Geometry check sheet. Reference: the model listing, model coordinates, mm. Face numbers are marked on the shaded views. A direction names the side the tool comes from. Round coordinates to 2 decimals unless told otherwise and drop trailing zeros. Write each loop counter-clockwise with the first axis right and the second up, starting at its lowest first coordinate (ties: lowest second). Pieces come first, ordered by that corner, then holes. Notation, with made-up numbers: (75, -23) -> (129, -23) arc R20 ccw to (129, 9) -> close; hole circle Ø9 at (59.5, 30). An arc over 180 degrees is marked (long way). Use a Markdown table: item, result.
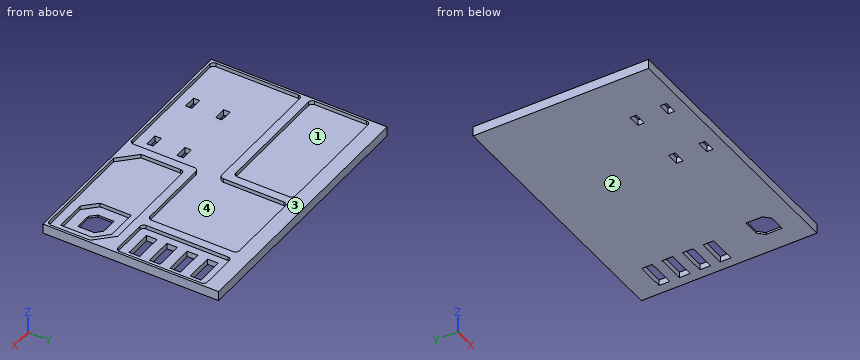
Autodesk Fusion 360 part; units mm, degrees
sketch "Sketch1" plane through (0, 0, 0) normal (0, 0, 1) x (1, 0, 0)
  line L0 (0, 0) -> (70.4, 0)
  line L1 (70.4, 0) -> (70.4, 46.4)
  line L2 (70.4, 46.4) -> (0, 46.4)
  line L3 (0, 46.4) -> (0, 0)
  line L4 (1.1, 1.1) -> (69.3, 1.1) construction
  line L5 (69.3, 1.1) -> (69.3, 45.3) construction
  line L6 (69.3, 45.3) -> (1.1, 45.3) construction
  line L7 (1.1, 45.3) -> (1.1, 1.1) construction
  line L8 (35.2, 45.3) -> (35.2, 1.1) construction
  line L9 (1.1, 23.2) -> (35.2, 23.2) construction
  line L10 (35.2, 23.2) -> (69.3, 23.2) construction
  line L11 (35.2, 45.3) -> (35.2, 42) construction
  line L12 (35.2, 42) -> (35, 42) construction
  line L13 (35, 42) -> (1.1, 42) construction
  line L14 (35.2, 42) -> (69.3, 42) construction
  line L15 (68.3, 42) -> (59.3, 42)
  line L16 (58.3, 41) -> (58.3, 19.9)
  line L17 (59.3, 18.9) -> (68.3, 18.9)
  line L18 (69.3, 19.9) -> (69.3, 41)
  line L19 (58.3, 30.45) -> (56.1, 30.45) construction
  line L20 (36.2, 42) -> (55.1, 42)
  line L21 (56.1, 41) -> (56.1, 19.9)
  line L22 (55.1, 18.9) -> (36.2, 18.9)
  line L23 (35.2, 30.45) -> (33, 30.45) construction
  line L24 (2.1, 42) -> (32, 42)
  line L25 (33, 41) -> (33, 27.6)
  line L26 (32, 26.6) -> (2.1, 26.6)
  line L27 (1.1, 27.6) -> (1.1, 41)
  line L28 (17.05, 26.6) -> (17.05, 24.4) construction
  line L29 (45.65, 18.9) -> (45.65, 16.7) construction
  line L30 (2.1, 1.1) -> (34.2, 1.1)
  line L31 (34.2, 24.3632) -> (2.1, 24.3632)
  line L32 (1.1, 23.3632) -> (1.1, 2.1)
  line L33 (35.2, 41) -> (35.2, 25.3632)
  line L34 (35.2, 17.9) -> (35.2, 2.1)
  line L35 (18.15, 24.3632) -> (18.15, 17.7632) construction
  line L36 (1.1, 1.1) -> (1.1, 2.2) construction
  line L37 (1.1, 1.1) -> (2.2, 1.1) construction
  line L38 (35.2, 1.1) -> (35.2, 2.2) construction
  line L39 (35.2, 1.1) -> (34.1, 1.1) construction
  line L40 (2.2, 2.2) -> (34.1, 2.2) construction
  line L41 (34.1, 2.2) -> (34.1, 17.7632) construction
  line L42 (34.1, 17.7632) -> (18.15, 17.7632) construction
  line L43 (2.2, 2.2) -> (2.2, 17.7632) construction
  line L44 (2.2, 17.7632) -> (18.15, 17.7632) construction
  line L45 (18.15, 2.2) -> (18.15, 17.7632) construction
  line L46 (18.15, 9.9816) -> (34.1, 9.9816) construction
  line L47 (18.15, 9.9816) -> (2.2, 9.9816) construction
  line L48 (10.175, 9.9816) -> (10.175, 11.0816) construction
  line L49 (18.15, 9.9816) -> (18.15, 17.7632) construction
  line L50 (18.15, 9.9816) -> (18.15, 2.2) construction
  line L51 (18.15, 13.8724) -> (17.05, 13.8724) construction
  line L52 (2.2, 2.2) -> (18.15, 2.2) construction
  line L53 (18.15, 2.2) -> (34.1, 2.2) construction
  line L54 (10.175, 2.2) -> (10.175, 3.3) construction
  line L55 (18.15, 6.0908) -> (17.05, 6.0908) construction
  line L56 (26.125, 2.2) -> (26.125, 3.3) construction
  line L57 (18.15, 6.0908) -> (19.25, 6.0908) construction
  line L58 (18.15, 13.8724) -> (19.25, 13.8724) construction
  line L59 (26.125, 9.9816) -> (26.125, 11.0816) construction
  line L60 (3.3, 16.6632) -> (17.05, 16.6632) construction
  line L61 (17.05, 16.6632) -> (17.05, 11.0816) construction
  line L62 (17.05, 11.0816) -> (3.3, 11.0816) construction
  line L63 (3.3, 11.0816) -> (3.3, 16.6632) construction
  line L64 (3.3, 8.8816) -> (17.05, 8.8816) construction
  line L65 (17.05, 8.8816) -> (17.05, 3.3) construction
  line L66 (17.05, 3.3) -> (3.3, 3.3) construction
  line L67 (3.3, 3.3) -> (3.3, 8.8816) construction
  line L68 (19.25, 8.8816) -> (33, 8.8816) construction
  line L69 (33, 8.8816) -> (33, 3.3) construction
  line L70 (33, 3.3) -> (19.25, 3.3) construction
  line L71 (19.25, 3.3) -> (19.25, 8.8816) construction
  line L72 (19.25, 16.6632) -> (33, 16.6632) construction
  line L73 (33, 16.6632) -> (33, 11.0816) construction
  line L74 (33, 11.0816) -> (19.25, 11.0816) construction
  line L75 (19.25, 11.0816) -> (19.25, 16.6632) construction
  line L76 (17.05, 11.0816) -> (17.05, 11.6316) construction
  line L77 (17.05, 11.0816) -> (16.5, 11.0816) construction
  line L78 (33, 11.0816) -> (33, 11.6316) construction
  line L79 (33, 11.0816) -> (32.45, 11.0816) construction
  line L80 (33, 3.3) -> (33, 3.85) construction
  line L81 (33, 3.3) -> (32.45, 3.3) construction
  line L82 (17.05, 3.3) -> (16.5, 3.3) construction
  line L83 (17.05, 3.3) -> (17.05, 3.85) construction
  line L84 (16.5, 11.6316) -> (13.2, 11.6316)
  line L85 (13.2, 11.6316) -> (13.2, 13.2816)
  line L86 (13.2, 13.2816) -> (16.5, 13.2816)
  line L87 (16.5, 13.2816) -> (16.5, 11.6316)
  line L88 (32.45, 11.6316) -> (29.15, 11.6316)
  line L89 (29.15, 11.6316) -> (29.15, 13.2816)
  line L90 (29.15, 13.2816) -> (32.45, 13.2816)
  line L91 (32.45, 13.2816) -> (32.45, 11.6316)
  line L92 (32.45, 3.85) -> (29.15, 3.85)
  line L93 (29.15, 3.85) -> (29.15, 5.5)
  line L94 (29.15, 5.5) -> (32.45, 5.5)
  line L95 (32.45, 5.5) -> (32.45, 3.85)
  line L96 (16.5, 3.85) -> (13.2, 3.85)
  line L97 (13.2, 3.85) -> (13.2, 5.5)
  line L98 (13.2, 5.5) -> (16.5, 5.5)
  line L99 (16.5, 5.5) -> (16.5, 3.85)
  line L100 (35.2, 10) -> (37.4, 10) construction
  line L101 (37.4, 16.7) -> (69.3, 16.7) construction
  line L102 (69.3, 16.7) -> (64.9, 16.7) construction
  line L103 (69.3, 16.7) -> (69.3, 12.3) construction
  line L104 (64.9, 16.7) -> (69.3, 12.3)
  line L105 (37.4, 1.1) -> (37.4, 5.5) construction
  line L106 (37.4, 1.1) -> (41.8, 1.1) construction
  line L107 (37.4, 5.5) -> (41.8, 1.1)
  line L108 (37.4, 15.7) -> (37.4, 5.5)
  line L109 (38.4, 16.7) -> (64.9, 16.7)
  line L110 (69.3, 12.3) -> (69.3, 2.1)
  line L111 (68.3, 1.1) -> (41.8, 1.1)
  line L112 (67.1, 14.5) -> (65.5444, 12.9444) construction
  line L113 (65.5444, 12.9444) -> (67.1, 11.3887)
  line L114 (65.5444, 12.9444) -> (63.9887, 14.5)
  line L115 (67.1, 11.3887) -> (69.3, 11.4) construction
  line L116 (63.9887, 14.5) -> (64, 16.7) construction
  line L117 (67.1, 1.1) -> (67.1, 3.3) construction
  line L118 (67.1, 11.3887) -> (67.1, 3.3)
  line L119 (67.1, 3.3) -> (59.011, 3.3)
  line L120 (63.9887, 14.5) -> (55.8998, 14.5414)
  line L121 (55.8998, 14.5414) -> (55.8584, 6.4525)
  line L122 (55.8584, 6.4525) -> (59.011, 3.3)
  line L123 (58.6142, 7.5858) -> (60.1501, 6.05)
  line L124 (64.35, 6.05) -> (60.1501, 6.05)
  line L125 (64.35, 10.2496) -> (64.35, 6.05)
  line L126 (63.5998, 10.9998) -> (64.35, 10.2496)
  line L127 (63.5998, 10.9998) -> (62.8438, 11.7558)
  line L128 (62.8438, 11.7558) -> (58.6357, 11.7774)
  line L129 (58.6357, 11.7774) -> (58.6142, 7.5858)
  arc A0 (2.1, 42) -> (1.1, 41) centre (2.1, 41) ccw
  arc A1 (33, 41) -> (32, 42) centre (32, 41) ccw
  arc A2 (32, 26.6) -> (33, 27.6) centre (32, 27.6) ccw
  arc A3 (1.1, 27.6) -> (2.1, 26.6) centre (2.1, 27.6) ccw
  arc A4 (36.2, 42) -> (35.2, 41) centre (36.2, 41) ccw
  arc A5 (56.1, 41) -> (55.1, 42) centre (55.1, 41) ccw
  arc A6 (55.1, 18.9) -> (56.1, 19.9) centre (55.1, 19.9) ccw
  arc A7 (36.2, 18.9) -> (35.2, 17.9) centre (36.2, 17.9) ccw
  arc A8 (34.2, 1.1) -> (35.2, 2.1) centre (34.2, 2.1) ccw
  arc A9 (1.1, 2.1) -> (2.1, 1.1) centre (2.1, 2.1) ccw
  arc A10 (2.1, 24.3632) -> (1.1, 23.3632) centre (2.1, 23.3632) ccw
  arc A11 (34.2, 24.3632) -> (35.2, 25.3632) centre (34.2, 25.3632) ccw
  arc A12 (38.4, 16.7) -> (37.4, 15.7) centre (38.4, 15.7) ccw
  arc A13 (68.3, 1.1) -> (69.3, 2.1) centre (68.3, 2.1) ccw
  arc A14 (59.3, 42) -> (58.3, 41) centre (59.3, 41) ccw
  arc A15 (58.3, 19.9) -> (59.3, 18.9) centre (59.3, 19.9) ccw
  arc A16 (68.3, 18.9) -> (69.3, 19.9) centre (68.3, 19.9) ccw
  arc A17 (69.3, 41) -> (68.3, 42) centre (68.3, 41) ccw
  line L130 (58.3, 41) -> (69.3, 41) construction
  line L131 (58.3, 19.9) -> (69.3, 19.9) construction
  line L132 (63.8, 19.9) -> (63.8, 41) construction
  line L133 (60.225, 39.7375) -> (67.375, 39.7375)
  line L134 (67.375, 39.7375) -> (67.375, 36.9875)
  line L135 (67.375, 36.9875) -> (60.225, 36.9875)
  line L136 (60.225, 36.9875) -> (60.225, 39.7375)
  line L137 (63.8, 41) -> (63.8, 39.7375) construction
  line L138 (60.225, 31.7115) -> (60.225, 34.4615)
  line L139 (60.225, 34.4615) -> (67.375, 34.4615)
  line L140 (67.375, 31.7115) -> (60.225, 31.7115)
  line L141 (67.375, 34.4615) -> (67.375, 31.7115)
  line L142 (67.375, 26.4355) -> (60.225, 26.4355)
  line L143 (60.225, 26.4355) -> (60.225, 29.1855)
  line L144 (67.375, 29.1855) -> (67.375, 26.4355)
  line L145 (60.225, 29.1855) -> (67.375, 29.1855)
  line L146 (60.225, 21.1595) -> (60.225, 23.9095)
  line L147 (60.225, 23.9095) -> (67.375, 23.9095)
  line L148 (67.375, 21.1595) -> (60.225, 21.1595)
  line L149 (67.375, 23.9095) -> (67.375, 21.1595)
  line L150 (63.8, 36.9875) -> (63.8, 34.4615) construction
  line L151 (63.8, 31.7115) -> (63.8, 29.1855) construction
  line L152 (63.8, 26.4355) -> (63.8, 23.9095) construction
  line L153 (70.4, 33.0328) -> (68.4, 33.0328) construction
  line L154 (13.2, 4.675) -> (11.2, 4.675) construction
  line L155 (14.85, 3.85) -> (14.85, 1.85) construction
  line L156 (11.2, 1.85) -> (68.3, 1.85)
  line L157 (68.3, 1.85) -> (68.3, 42.6341)
  line L158 (68.3, 42.6341) -> (11.2, 42.6341)
  line L159 (11.2, 42.6341) -> (11.2, 1.85)
  point P0 (58.3, 42)
  point P1 (69.3, 18.9)
  point P2 (56.1, 42)
  point P3 (56.1, 18.9)
  point P4 (35.2, 18.9)
  point P5 (1.1, 26.6)
  dimension "d1" = 46.4
  dimension "d2" = 70.4
  dimension "d3" = -1.1
  dimension "d5" = 3.3
  dimension "d6" = 11
  dimension "d7" = 23.1
  dimension "d8" = 2.2
  dimension "d9" = 23.1
  dimension "d10" = 20.9
  dimension "d11" = 2.2
  dimension "d12" = 15.4
  dimension "d13" = 2.2
  dimension "d14" = 2.2
  dimension "d16" = 6.6
  dimension "d18" = 1.1
  dimension "d19" = 1.1
  dimension "d20" = 1.1
  dimension "d21" = 1.1
  dimension "d22" = 1.1
  dimension "d23" = 1.1
  dimension "d24" = 1.1
  dimension "d25" = 1.1
  dimension "d26" = 1.1
  dimension "d27" = 1.1
  dimension "d28" = 1.1
  dimension "d29" = 1.1
  dimension "d30" = 0.55
  dimension "d31" = 0.55
  dimension "d32" = 0.55
  dimension "d33" = 0.55
  dimension "d34" = 0.55
  dimension "d35" = 0.55
  dimension "d36" = 0.55
  dimension "d37" = 0.55
  dimension "d38" = 3.3
  dimension "d39" = 1.65
  dimension "d40" = 3.3
  dimension "d41" = 1.65
  dimension "d42" = 3.3
  dimension "d43" = 1.65
  dimension "d44" = 3.3
  dimension "d45" = 1.65
  dimension "d46" = 2.2
  dimension "d47" = 4.4
  dimension "d48" = 4.4
  dimension "d49" = 4.4
  dimension "d50" = 4.4
  dimension "d51" = 2.2
  dimension "d52" = 2.2
  dimension "d53" = 2.2
  dimension "d55" = 2.2
  dimension "d56" = 8.089
  dimension "d57" = 8.089
  dimension "d58" = 8.089
  dimension "d59" = -2.75
  dimension "d60" = 1
  dimension "d61" = 1
  dimension "d62" = 1
  dimension "d63" = 1
  dimension "d64" = 1
  dimension "d65" = 2.75
  dimension "d66" = 1.2625
  dimension "d67" = 7.15
  dimension "d68" = 2.75
  dimension "d69" = 7.15
  dimension "d70" = 2.75
  dimension "d71" = 7.15
  dimension "d72" = 2.75
  dimension "d73" = 7.15
  dimension "d74" = 2.526
  dimension "d75" = 2.526
  dimension "d76" = 2.526
  dimension "d93" = 2
  dimension "d94" = 2
  dimension "d95" = 2
extrude "Extrude1" add sketch "Sketch1" against normal blind 2.5 contours L0 L1 L2 L3 | L15 L16 L17 A14 A15 L157 | L18 A16 A17 L157 | L15 L16 L17 L20 L21 L22 L24 L25 L26 L31 L33 L34 L104 L107 L108 L109 A1 A2 A4 A5 A6 A7 A8 A11 A12 A14 A15 L156 L157 L158 L159 | L104 L107 L108 L109 A12 L156 L157 | L104 L107 L110 L111 A13 L156 L157 | L24 L26 L27 A0 A3 L159 | L24 L25 L26 A1 A2 L159 | L20 L21 L22 L31 L33 L34 A4 A5 A6 A7 A8 A11 L156 L159 | L30 L31 L32 A8 A9 A10 L156 L159 | L84 L85 L86 L87 | L88 L89 L90 L91 | L92 L93 L94 L95 | L96 L97 L98 L99 | L113 L114 L118 L119 L120 L121 L122 | L123 L124 L125 L126 L127 L128 L129 | L133 L134 L135 L136 | L138 L139 L140 L141 | L142 L143 L144 L145 | L146 L147 L148 L149
extrude "Extrude2" cut sketch "Sketch1" against normal blind 1 contours L15 L16 L17 A14 A15 L157 | L18 A16 A17 L157 | L104 L107 L108 L109 A12 L156 L157 | L104 L107 L110 L111 A13 L156 L157 | L24 L26 L27 A0 A3 L159 | L24 L25 L26 A1 A2 L159 | L20 L21 L22 L31 L33 L34 A4 A5 A6 A7 A8 A11 L156 L159 | L30 L31 L32 A8 A9 A10 L156 L159 | L84 L85 L86 L87 | L88 L89 L90 L91 | L92 L93 L94 L95 | L96 L97 L98 L99 | L113 L114 L118 L119 L120 L121 L122 | L123 L124 L125 L126 L127 L128 L129 | L133 L134 L135 L136 | L138 L139 L140 L141 | L142 L143 L144 L145 | L146 L147 L148 L149
extrude "Extrude3" cut sketch "Sketch1" against normal blind 2 contours L113 L114 L118 L119 L120 L121 L122 | L123 L124 L125 L126 L127 L128 L129
extrude "Extrude4" cut sketch "Sketch1" against normal blind 10 contours L84 L85 L86 L87 | L88 L89 L90 L91 | L92 L93 L94 L95 | L96 L97 L98 L99 | L123 L124 L125 L126 L127 L128 L129 | L133 L134 L135 L136 | L138 L139 L140 L141 | L142 L143 L144 L145 | L146 L147 L148 L149
extrude "Extrude5" cut 1 faces at (23.4667, 0, -0.8333) along direction (0, 1, 0) blind 0.5
extrude "Extrude6" cut 1 faces at (46.9333, 46.4, -0.8333) along direction (0, -1, 0) blind 0.5
extrude "Extrude7" cut 1 faces at (70.4, 15.6333, -0.8333) along direction (-1, 0, 0) blind 0.5
extrude "Extrude8" cut 1 faces at (0, 30.7667, -0.8333) along direction (1, 0, 0) blind 0.5
(1) Section check D-D on z = -0.55. State how many separate pieces and enclosed holes the cut face has, plus the area to 3 significant figures.
A:
| item | result |
|---|---|
| separate pieces | 1 |
| enclosed holes | 4 |
| area | 654 mm2 |
(2) Section check B-B on x = 39.5. Record the cut outline in (y, z).
A:
| item | result |
|---|---|
| outline | (0.5, -2.5) -> (45.9, -2.5) -> (45.9, 0) -> (42, 0) -> (42, -1) -> (18.9, -1) -> (18.9, 0) -> (16.7, 0) -> (16.7, -1) -> (3.4, -1) -> (3.4, 0) -> (0.5, 0) -> close |
(3) Thickness scan on line 1 (Y direction, x = 46, z = -0.3); line 2 (X direction, y = 6, z = -0.3); line 3 (Y direction, x = 15.5, z = -1.25). Record the ranges inside material, lowest first.
A:
| item | result |
|---|---|
| line 1 | y = 0.5 to 1.1, 16.7 to 18.9, 42 to 45.9 |
| line 2 | x = 0.5 to 1.1, 35.2 to 37.4, 69.3 to 69.9 |
| line 3 | y = 0.5 to 3.85, 5.5 to 11.63, 13.28 to 45.9 |
(4) Section check C-C on y = 30. Record the cut outline in (x, z).
A:
| item | result |
|---|---|
| outline | (0.5, -2.5) -> (69.9, -2.5) -> (69.9, 0) -> (69.3, 0) -> (69.3, -1) -> (58.3, -1) -> (58.3, 0) -> (56.1, 0) -> (56.1, -1) -> (35.2, -1) -> (35.2, 0) -> (33, 0) -> (33, -1) -> (1.1, -1) -> (1.1, 0) -> (0.5, 0) -> close |
(5) Gauge pin test, flat ends, axial feed: pin 1 Ø4 at (x, y) = (44, 10.5) entering from +Z; pin 2 Ø3.5 at (x, y) = (64, 7.5) entering from +Z. Record the tip position at first contact, or that the pin passes through.
A:
| item | result |
|---|---|
| pin 1 | stops at z = -1 |
| pin 2 | stops at z = -2 |
(6) Section check A-A on y = 38.5. Record the cut outline in (x, z) (3 decimals), plus the area to 3 significant figures.
A:
| item | result |
|---|---|
| outline | (0.5, -2.5) -> (60.225, -2.5) -> (60.225, -1) -> (58.3, -1) -> (58.3, 0) -> (56.1, 0) -> (56.1, -1) -> (35.2, -1) -> (35.2, 0) -> (33, 0) -> (33, -1) -> (1.1, -1) -> (1.1, 0) -> (0.5, 0) -> close; (67.375, -2.5) -> (69.9, -2.5) -> (69.9, 0) -> (69.3, 0) -> (69.3, -1) -> (67.375, -1) -> close |
| area | 99.0 mm2 |
(7) Access from +Z, -Z, +X, -X, +Y, -Y to the whole of each face (thin tool, end or side, straight path). Record for the marked faces 1 and 2.
A:
| item | result |
|---|---|
| face 1 | +Z |
| face 2 | -Z, +X, -X, +Y, -Y |
(8) Release check for a two-part mould opening along X. For the marked faces 3 and 4 record: +X half, -X half, draft (parallel to the pull), parting line (faces both ways), or undercut.
A:
| item | result |
|---|---|
| face 3 | draft |
| face 4 | undercut |
